Here's how the part is built. I have some questions about the finished solid (model axes, mm). Face numbers are marked on the shaded views. A direction names the side the tool comes from. Give positions to 0.01 mm unless a question says otherwise; leave off trailing zeros. Write each loop counter-clockwise with the first axis right and the second up, starting at its lowest first coordinate (ties: lowest second). Pieces come first, ordered by that corner, then holes. Notation, with made-up numbers: (27.25, -13) -> (61.25, -13) arc R23 cw to (61.25, 13) -> close; hole circle Ø5 at (51, 87). An arc over 180 degrees is marked (long way). Answer as CSV lines item,"result". Start each with the question number.
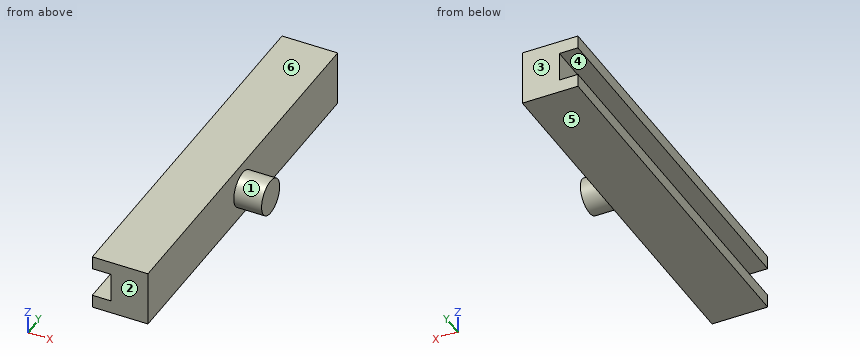
from build123d import *

# Parameters (mm, degrees)
BOSS_EXTRUDE1_DEPTH = 40
SKETCH3_R           = 1.905
BOSS_EXTRUDE2_DEPTH = 3


with BuildPart() as part:
    # Sketch2 → Boss-Extrude1 (new body)
    with BuildSketch(Plane(origin=(0, 0, 0), x_dir=(1, 0, 0), z_dir=(0, 1, 0))):
        Polygon((0, 0), (6, 0), (6, 6), (0, 6), (0, 4.5875), (2, 4.5875), (2, 1.4125), (0, 1.4125), align=None)
    extrude(amount=-BOSS_EXTRUDE1_DEPTH)

    # Sketch3 → Boss-Extrude2 (add)
    with BuildSketch(Plane(origin=(6, 0, 0), x_dir=(0, 0, -1), z_dir=(1, 0, 0))):
        with Locations((3, -20)):
            Circle(SKETCH3_R)
    extrude(amount=BOSS_EXTRUDE2_DEPTH)


solid = part.part
Item 1: I'm going to push flat-ended pins straight in: pin 1 (1.5 mm diameter, centred on x = 8, z = -2.5, fed in from -Y) (3 decimals); pin 2 (1 mm diameter, centred on x = 7, y = -28.5, fed in from -Z); pin 3 (1 mm diameter, centred on y = -16, z = -4, fed in from -X). Where does each tip first touch, or does it pass through?
Item 2: We'd pull the mould along Z, two halves only. Please class the marked faces 3, 4, 5 and 6: released by +Z, released by -Z, zero draft, split by the parting line, or undercut.
Item 3: If I drill on line 1 (X direction, y = -27, z = -2.05); line 2 (X direction, y = -36.5, z = -0.7); line 3 (Z direction, x = 8.25, y = -21), over which ranges is the centre line in solid material (lowest first)? Write a range as [from, to].
Item 4: For the marked faces 1 and 2, which set-ups out of +Z, -Z, +X, -X, +Y, -Y let a thin tool reach every point of the face, with its end or its side?
Item 5: If we section it at C-C (y = -4): Please give me the cut outline in (x, z), and give its area (4 significant figures).
Item 6: If we section it at D-D (z = -5.45): Please give me the cut outline in (x, y).
Item 7: If we section it at B-B (z = -3): Please give me the cut outline in (x, y) (3 decimals), and give its area (3 significant figures).
Item 8: If we section it at A-A (x = 1.25): Please give me the cut outline in (y, z), and give its area (3 significant figures).
Final values:
1,pin 1,"y = -21.905"
1,pin 2,"through"
1,pin 3,"x = 2"
2,face 3,"zero draft"
2,face 4,"undercut"
2,face 5,"released by -Z"
2,face 6,"released by +Z"
3,line 1,"[2, 6]"
3,line 2,"[0, 6]"
3,line 3,"[-4.62, -1.38]"
4,face 1,"+X"
4,face 2,"+Z, -Z, +X, -X, -Y"
5,outline,"(0, -6) -> (6, -6) -> (6, 0) -> (0, 0) -> (0, -1.41) -> (2, -1.41) -> (2, -4.59) -> (0, -4.59) -> close"
5,area,"29.65 mm2"
6,outline,"(0, -40) -> (6, -40) -> (6, 0) -> (0, 0) -> close"
7,outline,"(2, -40) -> (6, -40) -> (6, -21.905) -> (9, -21.905) -> (9, -18.095) -> (6, -18.095) -> (6, 0) -> (2, 0) -> close"
7,area,"171 mm2"
8,outline,"(-40, -6) -> (0, -6) -> (0, -4.59) -> (-40, -4.59) -> close; (-40, -1.41) -> (0, -1.41) -> (0, 0) -> (-40, 0) -> close"
8,area,"113 mm2"
